from build123d import *
from OCP.BRepFilletAPI import BRepFilletAPI_MakeChamfer

# Parameters (mm, degrees)
SCHIZZO1_W                   = 34
SCHIZZO1_H                   = 30
ESTRUSIONE_ESTRUSIONE1_DEPTH = 22
SCHIZZO2_W                   = 1
SCHIZZO2_H                   = 14.267949192
TAGLIO_ESTRUSIONE1_DEPTH     = 37.193922142
SCHIZZO3_W                   = 10.8571
SCHIZZO3_H                   = 4
TAGLIO_ESTRUSIONE2_DEPTH     = 37.193922142
SCHIZZO4_W                   = 11.8571
SCHIZZO4_H                   = 4
TAGLIO_ESTRUSIONE3_DEPTH     = 37.193922142
SCHIZZO5_W                   = 1
SCHIZZO5_H                   = 10.267949192
TAGLIO_ESTRUSIONE4_DEPTH     = 37.193922142
SCHIZZO6_W                   = 15.2
SCHIZZO6_H                   = 0.4
TAGLIO_ESTRUSIONE5_DEPTH     = 37.193922142
SFORMO1_ANGLE                = 60
SFORMO2_ANGLE                = 60
SFORMO3_ANGLE                = 45
SFORMO4_ANGLE                = 45
SMUSSO1_SIZE                 = 0.230940108
SMUSSO1_SIZE2                = 0.4
SMUSSO2_SIZE                 = 0.379
SMUSSO3_SIZE                 = 1
SCHIZZO13_W                  = 7.577824215
SCHIZZO13_H                  = 21.931685432
TAGLIO_ESTRUSIONE6_DEPTH     = 37.193922142


with BuildPart() as part:
    # Schizzo1 → Estrusione-Estrusione1 (new body)
    with BuildSketch(Plane(origin=(0, 11, 0), x_dir=(1, 0, 0), z_dir=(0, 1, 0))):
        with Locations((0, -15)):
            Rectangle(SCHIZZO1_W, SCHIZZO1_H)
    extrude(amount=-ESTRUSIONE_ESTRUSIONE1_DEPTH)

    # Schizzo2 → Taglio-Estrusione1 (cut, through all)
    with BuildSketch(Plane.XY.offset(30)):
        with Locations((16.5, -3.866025404)):
            Rectangle(SCHIZZO2_W, SCHIZZO2_H)
    extrude(amount=-TAGLIO_ESTRUSIONE1_DEPTH, mode=Mode.SUBTRACT)

    # Schizzo3 → Taglio-Estrusione2 (cut, through all)
    with BuildSketch(Plane.XY.offset(30)):
        with Locations((10.57145, -9)):
            Rectangle(SCHIZZO3_W, SCHIZZO3_H)
    extrude(amount=-TAGLIO_ESTRUSIONE2_DEPTH, mode=Mode.SUBTRACT)

    # Schizzo4 → Taglio-Estrusione3 (cut, through all)
    with BuildSketch(Plane.XY.offset(30)):
        with Locations((-11.07145, -9)):
            Rectangle(SCHIZZO4_W, SCHIZZO4_H)
    extrude(amount=-TAGLIO_ESTRUSIONE3_DEPTH, mode=Mode.SUBTRACT)

    # Schizzo5 → Taglio-Estrusione4 (cut, through all)
    with BuildSketch(Plane.XY.offset(30)):
        with Locations((-16.5, -1.866025404)):
            Rectangle(SCHIZZO5_W, SCHIZZO5_H)
    extrude(amount=-TAGLIO_ESTRUSIONE4_DEPTH, mode=Mode.SUBTRACT)

    # Schizzo6 → Taglio-Estrusione5 (cut, through all)
    with BuildSketch(Plane.XY.offset(30)):
        with Locations((0, 10.8)):
            Rectangle(SCHIZZO6_W, SCHIZZO6_H)
    extrude(amount=-TAGLIO_ESTRUSIONE5_DEPTH, mode=Mode.SUBTRACT)

    # Sformo1
    sformo1_faces = [part.faces().sort_by_distance(p)[0] for p in [
        (16.5, 3.267949192, 15),
    ]]
    draft(sformo1_faces, Plane(origin=(16, 3.267949192, 0), x_dir=(0, 0, 1), z_dir=(1, 0, 0)), SFORMO1_ANGLE)

    # Sformo2
    sformo2_faces = [part.faces().sort_by_distance(p)[0] for p in [
        (-16.5, 3.267949192, 15),
    ]]
    draft(sformo2_faces, Plane(origin=(-16, -7, 0), x_dir=(0, 0, -1), z_dir=(-1, 0, 0)), SFORMO2_ANGLE)

    # Sformo3
    sformo3_faces = [part.faces().sort_by_distance(p)[0] for p in [
        (5.1429, -9, 15),
        (-5.1429, -9, 15),
    ]]
    draft(sformo3_faces, Plane(origin=(0, -11, 0), x_dir=(0, 0, -1), z_dir=(0, -1, 0)), SFORMO3_ANGLE)

    # Sformo4
    sformo4_faces = [part.faces().sort_by_distance(p)[0] for p in [
        (-7.6, 10.8, 15),
        (7.6, 10.8, 15),
    ]]
    draft(sformo4_faces, Plane(origin=(-7.6, 10.6, 0), x_dir=(1, 0, 0), z_dir=(0, 1, 0)), SFORMO4_ANGLE)

    # Schizzo7 → Taglia-Rivoluzione1 (revolve, cut)
    with BuildSketch(Plane.XZ, mode=Mode.PRIVATE) as taglia_rivoluzione1_sk:
        Polygon((7.5, 30), (0, 30), (0, 0), (7.5, 0), (7.5, 2), (7.85, 2), (7.85, 3.15), (7.5, 3.15), (7.5, 26.85), (7.85, 26.85), (7.85, 28), (7.5, 28), align=None)
    revolve(taglia_rivoluzione1_sk.sketch.rotate(Axis((0, 0, 30), (0, 0, -1)), 180), axis=Axis((0, 0, 30), (0, 0, -1)), mode=Mode.SUBTRACT)

    # Schizzo8 → Taglia-Rivoluzione2 (revolve, cut)
    with BuildSketch(Plane.XY.offset(6), mode=Mode.PRIVATE) as taglia_rivoluzione2_sk:
        Polygon((-10.379, 11), (-12, 11), (-12, -7), (-10.3, -7), (-10.3, 3), (-10.379, 3), align=None)
    revolve(taglia_rivoluzione2_sk.sketch.rotate(Axis((-12, 11, 6), (0, -1, 0)), 270), axis=Axis((-12, 11, 6), (0, -1, 0)), mode=Mode.SUBTRACT)

    # Schizzo9 → Taglia-Rivoluzione3 (revolve, cut)
    with BuildSketch(Plane.XY.offset(24), mode=Mode.PRIVATE) as taglia_rivoluzione3_sk:
        Polygon((-10.379, 11), (-12, 11), (-12, -7), (-10.3, -7), (-10.3, 3), (-10.379, 3), align=None)
    revolve(taglia_rivoluzione3_sk.sketch.rotate(Axis((-12, 11, 24), (0, -1, 0)), 270), axis=Axis((-12, 11, 24), (0, -1, 0)), mode=Mode.SUBTRACT)

    # Schizzo10 → Taglia-Rivoluzione4 (revolve, cut)
    with BuildSketch(Plane.XY.offset(6), mode=Mode.PRIVATE) as taglia_rivoluzione4_sk:
        Polygon((13.621, 11), (12, 11), (12, -7), (13.7, -7), (13.7, 3), (13.621, 3), align=None)
    revolve(taglia_rivoluzione4_sk.sketch.rotate(Axis((12, 11, 6), (0, -1, 0)), 270), axis=Axis((12, 11, 6), (0, -1, 0)), mode=Mode.SUBTRACT)

    # Schizzo11 → Taglia-Rivoluzione5 (revolve, cut)
    with BuildSketch(Plane.XY.offset(24), mode=Mode.PRIVATE) as taglia_rivoluzione5_sk:
        Polygon((13.621, 11), (12, 11), (12, -7), (13.7, -7), (13.7, 3), (13.621, 3), align=None)
    revolve(taglia_rivoluzione5_sk.sketch.rotate(Axis((12, 11, 24), (0, -1, 0)), 270), axis=Axis((12, 11, 24), (0, -1, 0)), mode=Mode.SUBTRACT)

    # Smusso1: one chamfer whose edges measure the first distance from different faces: ONE call of the kernel's chamfer builder (chamfer() names one face for all edges)
    smusso1_edges_1 = [part.edges().sort_by_distance(p)[0] for p in [
        (-12, -7, 7.7),
        (-12, -7, 25.7),
    ]]
    smusso1_side_1 = [part.faces().sort_by_distance(p)[0] for p in [
        (-12.626775869, -7, 15),
    ]]
    smusso1_edges_2 = [part.edges().sort_by_distance(p)[0] for p in [
        (12, -7, 7.7),
        (12, -7, 25.7),
    ]]
    smusso1_side_2 = [part.faces().sort_by_distance(p)[0] for p in [
        (12.626775869, -7, 15),
    ]]
    smusso1 = BRepFilletAPI_MakeChamfer(part.part.solid().wrapped)
    for e in smusso1_edges_1:
        smusso1.Add(SMUSSO1_SIZE, SMUSSO1_SIZE2, e.wrapped, smusso1_side_1[0].wrapped)  # the first distance lies on this face
    for e in smusso1_edges_2:
        smusso1.Add(SMUSSO1_SIZE, SMUSSO1_SIZE2, e.wrapped, smusso1_side_2[0].wrapped)  # the first distance lies on this face
    add(Compound.cast(smusso1.Shape()), mode=Mode.REPLACE)

    # Smusso2
    smusso2_edges = [part.edges().sort_by_distance(p)[0] for p in [
        (-12, 11, 7.621),
        (-12, 11, 25.621),
        (12, 11, 7.621),
        (12, 11, 25.621),
        (-12.5, 11, 30),
        (12.5, 11, 0),
        (-12.5, 11, 0),
        (12.5, 11, 30),
    ]]
    chamfer(smusso2_edges, length=SMUSSO2_SIZE)

    # Smusso3
    smusso3_edges = [part.edges().sort_by_distance(p)[0] for p in [
        (17, 11, 15),
        (-17, 11, 15),
    ]]
    chamfer(smusso3_edges, length=SMUSSO3_SIZE)

    # Schizzo13 → Taglio-Estrusione6 (cut, through all)
    with BuildSketch(Plane(origin=(0, 0, 0), x_dir=(-1, 0, 0), z_dir=(0, 0, -1))):
        with Locations((-16.788912107, 1.791699595)):
            Rectangle(SCHIZZO13_W, SCHIZZO13_H)
    extrude(amount=-TAGLIO_ESTRUSIONE6_DEPTH, mode=Mode.SUBTRACT)


solid = part.part
CAD build for the part. Positions are in the model's coordinates, mm. A direction names the side the tool comes from. Give positions to 0.01 mm unless a question says otherwise; leave off trailing zeros. Loops run counter-clockwise (first coordinate to the right, second up) from the corner with the lowest first, then second, coordinate; pieces in that order, holes last. Notation, with made-up numbers: M 64.5,25 L 82.5,25 A24 ccw 82.5,39 Z; hole C 68.25,-18.5 d6. An arc over 180 degrees is marked long. One line per question, with ' | ' between items. Start each with the question number.
1. Saw through at A-A on z = 24. State how many separate pieces and enclosed holes the cut face has, plus the area to 3 significant figures.
2. Saw through at D-D on z = 17. Give the cut face in (x, y).
3. Two-plate mould, pull along Z, no slides. Class faces 4 (the face through (-13.03, -1.73, 7.35)), 5 (the face through (10.38, 6.86, 24.05)), 6 (the face through (10, 11, 15)): pulls with the +Z half, pulls with the -Z half, needs draft (parallel to the pull), parting line crosses it, or undercut.
4. Flat gauge pins, fed straight in: pin 1 (12 mm diameter, centred on x = -1, z = 13, fed in from +Y); pin 2 (1.5 mm diameter, centred on x = -12, z = 9, fed in from -Y); pin 3 (7.5 mm diameter, centred on x = -12.5, z = 20, fed in from -Y). Where does each tip first touch, or does it go through?
5. 3-axis set-ups, long thin cutter, end or side, ignore diameter. For faces 1 (the face through (0, -11, 15)), 2 (the face through (10.3, -1.73, 6.05)), 3 (the face through (-16, -2, 15)): which of +Z, -Z, +X, -X, +Y, -Y reach the whole face in a straight line?
6. Probe L1, parallel to Z at x = 12, y = 1; L2, parallel to Y at x = 0, z = 27.3; L3, parallel to X at y = -0.25, z = 24. List the from-to ranges inside material, lowest first. Write a range as from..to.
Result sheet:
1) separate pieces: 2 | enclosed holes: 1 | area: 294 mm^2
2) outline: M -17,5 L -16,3.27 L -16,-7 L -9.14,-7 L -5.14,-11 L 5.14,-11 L 9.14,-7 L 13,-7 L 13,11 L 8,11 L 7.6,10.6 L -7.6,10.6 L -8,11 L -16,11 L -17,10 Z; hole C 0,0 d15
3) face 4: undercut | face 5: undercut | face 6: needs draft
4) pin 1: stops at y = 10.6 | pin 2: stops at y = -7 | pin 3: stops at y = -7.39
5) face 1: +Z, -Z, +X, -X, -Y | face 2: -Y | face 3: +Z, -Z, -X, -Y
6) L1: z = 0..4.3, 7.7..22.3, 25.7..30 | L2: y = -11..-7.85, 7.85..10.6 | L3: x = -16..-13.7, -10.3..-7.5, 7.5..10.3
